```python
from build123d import *

# Parameters (mm, degrees)
BOSS_EXTRUDE1_DEPTH     = 3
SKETCH2_W               = 106.5
SKETCH2_H               = 106.5
CUT_EXTRUDE1_DEPTH      = 0.5
SKETCH4_W               = 8
SKETCH4_H               = 3
CUT_EXTRUDE2_DEPTH      = 105.126526789
CIRPATTERN1_START       = -24.999999535
CIRPATTERN1_OUTLINE_W   = 3
CIRPATTERN1_OUTLINE_H   = 3
CIRPATTERN1_DEPTH       = 8
CIRPATTERN1_START_2     = 16.999999535
CIRPATTERN1_2_OUTLINE_W = 3
CIRPATTERN1_2_OUTLINE_H = 3
CIRPATTERN1_2_DEPTH     = 8
CIRPATTERN1_3_DEPTH     = 8
CIRPATTERN1_4_DEPTH     = 8


# Read off the part's stored shape, not the designer's step: CirPattern1
with BuildPart() as part:
    # Sketch1 → Boss-Extrude1 (new body)
    with BuildSketch(Plane(origin=(0, 0, 0), x_dir=(1, 0, 0), z_dir=(0, 1, 0))):
        Polygon((-25.000000465, 72.168783917), (24.999999535, 72.168783917), (75.000001394, -14.433756462), (49.999999071, -57.735027455), (-50, -57.735027455), (-75.000000465, -14.433756462), align=None)
    extrude(amount=BOSS_EXTRUDE1_DEPTH)

    # Sketch2 → Cut-Extrude1 (cut)
    with BuildSketch(Plane(origin=(0, 3, 0), x_dir=(1, 0, 0), z_dir=(0, 1, 0))):
        Rectangle(SKETCH2_W, SKETCH2_H)
    extrude(amount=-CUT_EXTRUDE1_DEPTH, mode=Mode.SUBTRACT)

    # Sketch4 → Cut-Extrude2 (cut, through all)
    with BuildSketch(Plane.XZ):
        with Locations((20.999999535, -70.668783917)):
            Rectangle(SKETCH4_W, SKETCH4_H)
    cut_extrude2 = extrude(amount=-CUT_EXTRUDE2_DEPTH, mode=Mode.SUBTRACT)

    # Mirror1: Cut-Extrude2 across plane
    add(cut_extrude2.mirror(Plane(origin=(0, 0, 0), x_dir=(0, 0, 1), z_dir=(1, 0, 0))), mode=Mode.SUBTRACT)

    # CirPattern1 outline → CirPattern1 (cut)
    with BuildSketch(Plane(origin=(0, 0, 0), x_dir=(0.8660254037844362, 0, -0.5000000000000042), z_dir=(0.5000000000000042, 0, 0.8660254037844363)).offset(CIRPATTERN1_START)):
        with Locations((-70.668783917, 1.5)):
            Rectangle(CIRPATTERN1_OUTLINE_W, CIRPATTERN1_OUTLINE_H)
    extrude(amount=CIRPATTERN1_DEPTH, mode=Mode.SUBTRACT)

    # CirPattern1 2 outline → CirPattern1 2 (cut)
    with BuildSketch(Plane(origin=(0, 0, 0), x_dir=(0.8660254037844362, 0, -0.5000000000000042), z_dir=(0.5000000000000042, 0, 0.8660254037844363)).offset(CIRPATTERN1_START_2)):
        with Locations((-70.668783917, 1.5)):
            Rectangle(CIRPATTERN1_2_OUTLINE_W, CIRPATTERN1_2_OUTLINE_H)
    extrude(amount=CIRPATTERN1_2_DEPTH, mode=Mode.SUBTRACT)

    # CirPattern1 3 outline → CirPattern1 3 (cut)
    with BuildSketch(Plane(origin=(0, 0, 0), x_dir=(0.8660254037844431, 0, 0.4999999999999921), z_dir=(0.4999999999999921, 0, -0.8660254037844433)).offset(CIRPATTERN1_START)):
        Polygon((69.168783917, -3), (72.168784721, -3), (72.168784587, 0), (69.168783917, 0), align=None)
    extrude(amount=CIRPATTERN1_3_DEPTH, mode=Mode.SUBTRACT)

    # CirPattern1 4 outline → CirPattern1 4 (cut)
    with BuildSketch(Plane(origin=(0, 0, 0), x_dir=(0.8660254037844431, 0, 0.4999999999999921), z_dir=(0.4999999999999921, 0, -0.8660254037844433)).offset(CIRPATTERN1_START_2)):
        Polygon((69.168783917, -3), (72.168784721, -3), (72.168784587, 0), (69.168783917, 0), align=None)
    extrude(amount=CIRPATTERN1_4_DEPTH, mode=Mode.SUBTRACT)


solid = part.part
```
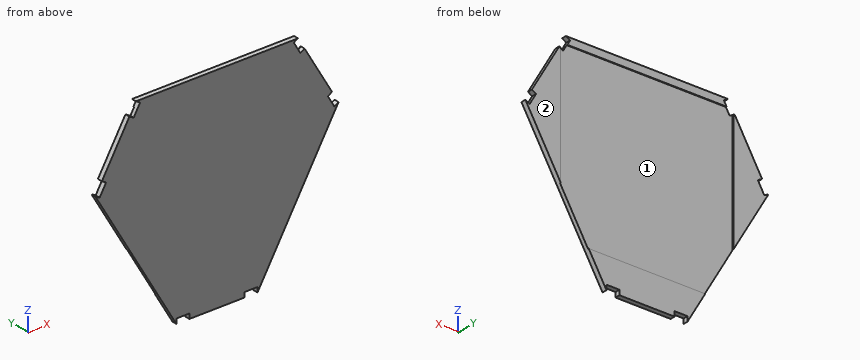
Source: CAD feature listing. Evaluate the final solid. Frame: model axes, mm. Face numbers are marked on the shaded views. Round coordinates to 2 decimals unless told otherwise and drop trailing zeros. Order: outer loops, then holes, each group sorted by start corner. A loop starts at its lowest first (then second) coordinate and runs counter-clockwise, first axis right, second up. Notation, with made-up numbers: (-32, -15) -> (-1, -15) arc R18 cw to (-1, -10) -> close; hole circle Ø10 at (11, 72.5). An arc over 180 degrees is marked (long way). Use CSV: the item, a comma, the result in double quotes.
(1) Section D-D on x = -42.5. Return the cut outline in (y, z), and give its area (3 significant figures).
Report:
outline,"(0, -41.86) -> (2.5, -41.86) -> (2.5, 53.25) -> (3, 53.25) -> (3, 57.74) -> (0, 57.74) -> close"
area,"251 mm^2"
(2) First-contact query: pin 1 Ø0.6 at (x, y) = (-17.5, 3) entering from -Z; pin 2 Ø1.5 at (y, z) = (1, -70) entering from -X; pin 3 Ø0.9 at (y, z) = (2, -71) entering from +X. Flat tips, straight axial feed; report the tip coordinate or a pass-through.
Report:
pin 1,"z = -69.17"
pin 2,"x = -26.69"
pin 3,"x = 25.93"
(3) Ray query, L1, parallel to Y at x = 34.5, z = -10; L2, parallel to X at y = 1.1, z = 49.5; L3, parallel to Z at x = -22, y = 2.1. Return the intervals inside material, ascending.
Report:
L1,"0 to 2.5"
L2,"-54.75 to -51.74, -51.29 to 51.29, 51.74 to 54.75"
L3,"-69.17 to 57.74"
(4) Section C-C on z = 40.5. Return the cut outline in (x, y), and give its area (3 significant figures).
Report:
outline,"(-59.95, 0) -> (59.95, 0) -> (59.95, 3) -> (53.25, 3) -> (53.25, 2.5) -> (-53.25, 2.5) -> (-53.25, 3) -> (-59.95, 3) -> close"
area,"306 mm^2"
(5) Section B-B on x = -4.5. Return the cut outline in (y, z), and give its area (3 significant figures).
Report:
outline,"(0, -72.17) -> (3, -72.17) -> (3, -53.25) -> (2.5, -53.25) -> (2.5, 53.25) -> (3, 53.25) -> (3, 57.74) -> (0, 57.74) -> close"
area,"336 mm^2"
(6) Pull-direction query (Z, two-part tool) for the marked faces 1 and 2; classes: +Z half, -Z half, draft (parallel to the pull), parting line (faces both ways), or undercut.
Report:
face 1,"undercut"
face 2,"draft"
